from build123d import *

# Parameters (mm, degrees)
SKETCH_W      = 31
SKETCH_H      = 135.1
PAD_DEPTH     = 217.3
SKETCH001_R   = 8
SKETCH001_R_2 = 10
PAD001_DEPTH  = 5.2
SKETCH002_R   = 4
POCKET_DEPTH  = 5


with BuildPart() as part:
    # Sketch → Pad (new body)
    with BuildSketch(Plane.XY):
        with Locations((15.5, 67.55)):
            Rectangle(SKETCH_W, SKETCH_H)
    extrude(amount=PAD_DEPTH)

    # Sketch001 (on Face6 of Pad) → Pad001 (join)
    with BuildSketch(Plane.XY.offset(217.3)):
        with Locations((15.5, 33.8)):
            Circle(SKETCH001_R)
        with Locations((15.5, 67.55)):
            Circle(SKETCH001_R_2)
        with Locations((15.5, 101.3)):
            Circle(SKETCH001_R)
    extrude(amount=PAD001_DEPTH)

    # Sketch002 (on Face11 of Pad001) → Pocket (cut)
    with BuildSketch(Plane.XY.offset(222.5)):
        with Locations((15.5, 101.3)):
            Circle(SKETCH002_R)
        with Locations((15.5, 33.8)):
            Circle(SKETCH002_R)
    extrude(amount=-POCKET_DEPTH, mode=Mode.SUBTRACT)


solid = part.part
For this review, take the finished solid that the model builds, in its own axes (mm). A direction names the side the tool comes from. Coordinates: 2 decimals unless noted, no trailing zeros. Write each loop counter-clockwise with the first axis right and the second up, starting at its lowest first coordinate (ties: lowest second). Pieces come first, ordered by that corner, then holes. Notation, with made-up numbers: (32, 36) -> (60, 36) arc R21 cw to (60, 60) -> close; hole circle Ø4 at (-29.75, 62.5). An arc over 180 degrees is marked (long way). Write each question's results on one line, items separated by ' | '. Start each with the question number.
1) Consider section C-C (y = 20). Write out the cut boundary in (x, z).
2) For faces 4 (the face through (13.33, 57.79, 219.86)), 5 (the face through (0, 67, 107)), list the 3-axis set-ups (+Z, -Z, +X, -X, +Y, -Y) from which the entire face can be reached by the end or side of a thin tool; tool diameter is ignored.
3) The part is to be moulded in two halves that separate along Y. For faces 1 (the face through (15, 101, 217.5)), 2 (the face through (13.6, 105, 222.5)), 3 (the face through (15, 0, 107)), say which applies: +Y half, -Y half, draft (parallel to the pull), parting line (faces both ways), or undercut.
4) Consider section A-A (x = 15.5). Write out the cut boundary in (y, z), plus the area to 3 significant figures.
5) Consider section B-B (y = 33.8). Write out the cut boundary in (x, z).
6) Wall thickness on L1, parallel to Y at x = 15.5, z = 221.45; L2, parallel to X at y = 101, z = 219; L3, parallel to Z at x = 6.5, y = 113.5: over which ranges is each line inside the solid? List them lowest first. Write a range as [from, to].
7) Consider section D-D (x = 3). Write out the cut boundary in (y, z).
8) Insertion check: pin 1 (2 mm diameter, centred on x = 11.5, y = 87.5, fed in from +Z); pin 2 (6.5 mm diameter, centred on x = 15.5, y = 33.8, fed in from +Z). Each pin has a flat end and moves straight along its axis. Give the tip position at first contact, or say it passes through.
Geometry says:
1) outline: (0, 0) -> (31, 0) -> (31, 217.3) -> (0, 217.3) -> close
2) face 4: +Z | face 5: +Z, -Z, -X, +Y, -Y
3) face 1: undercut | face 2: draft | face 3: -Y half
4) outline: (0, 0) -> (135.1, 0) -> (135.1, 217.3) -> (109.3, 217.3) -> (109.3, 222.5) -> (105.3, 222.5) -> (105.3, 217.5) -> (97.3, 217.5) -> (97.3, 222.5) -> (93.3, 222.5) -> (93.3, 217.3) -> (77.55, 217.3) -> (77.55, 222.5) -> (57.55, 222.5) -> (57.55, 217.3) -> (41.8, 217.3) -> (41.8, 222.5) -> (37.8, 222.5) -> (37.8, 217.5) -> (29.8, 217.5) -> (29.8, 222.5) -> (25.8, 222.5) -> (25.8, 217.3) -> (0, 217.3) -> close | area: 29,500 mm^2
5) outline: (0, 0) -> (31, 0) -> (31, 217.3) -> (23.5, 217.3) -> (23.5, 222.5) -> (19.5, 222.5) -> (19.5, 217.5) -> (11.5, 217.5) -> (11.5, 222.5) -> (7.5, 222.5) -> (7.5, 217.3) -> (0, 217.3) -> close
6) L1: [25.8, 29.8], [37.8, 41.8], [57.55, 77.55], [93.3, 97.3], [105.3, 109.3] | L2: [7.51, 11.51], [19.49, 23.49] | L3: [0, 217.3]
7) outline: (0, 0) -> (135.1, 0) -> (135.1, 217.3) -> (0, 217.3) -> close
8) pin 1: z = 217.3 | pin 2: z = 217.5
